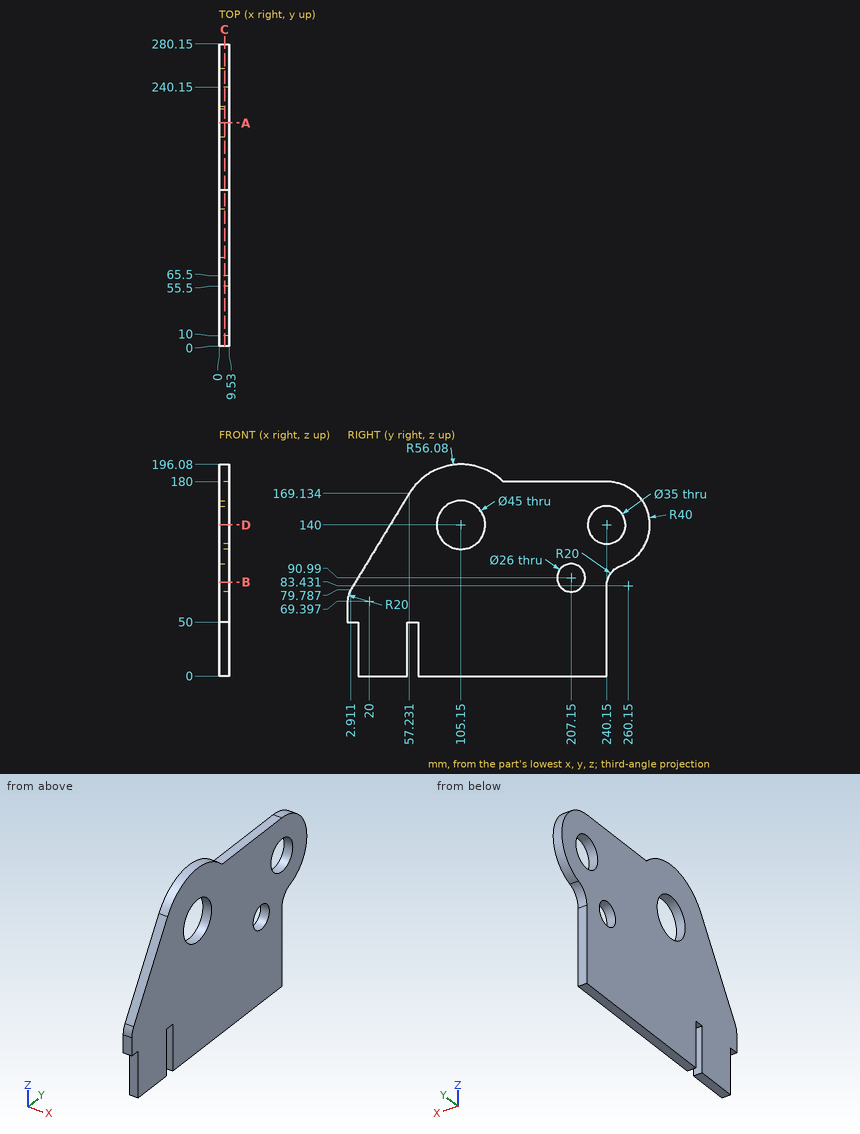
Answer from the drawing. Dimensions are ordinates in mm from the lowest x, y and z of the part. Coordinates: 2 decimals unless noted, no trailing zeros. Write each loop counter-clockwise with the first axis right and the second up, starting at its lowest first coordinate (ties: lowest second). Pieces come first, ordered by that corner, then holes. Notation, with made-up numbers: M -30.75,61 L 21.25,61 A34 cw 21.25,94 Z; hole C 47.5,-10.75 d5. An arc over 180 degrees is marked long. Use a Markdown table: item, result.
Q1. The part is cut by section D-D, the plane z = 140. Write down the section's boundary in (x, y).
Answer block:
| item | result |
|---|---|
| outline | M 0,39.52 L 9.53,39.52 L 9.53,82.65 L 0,82.65 Z; M 0,127.65 L 9.53,127.65 L 9.53,222.65 L 0,222.65 Z; M 0,257.65 L 9.53,257.65 L 9.53,280.15 L 0,280.15 Z |
Q2. Each of these flat-tipped pins is pushed along its axis until it touches: pin 1 Ø4 at (x, z) = (8, 164) entering from +Y; pin 2 Ø5 at (x, y) = (4.5, 61.5) entering from -Z; pin 3 Ø5 at (x, z) = (5, 25) entering from +Y. Where does it stop, or does it pass through?
Answer block:
| item | result |
|---|---|
| pin 1 | stops at y = 273.56 |
| pin 2 | stops at z = 50 |
| pin 3 | stops at y = 240.15 |
Q3. The part is cut by section A-A, the plane y = 207.15. Write down the section's boundary in (x, z), then the cut area to 3 significant figures.
Answer block:
| item | result |
|---|---|
| outline | M 0,0 L 9.53,0 L 9.53,77.99 L 0,77.99 Z; M 0,103.99 L 9.53,103.99 L 9.53,180 L 0,180 Z |
| area | 1,470 mm2 |
Q4. The part is cut by section C-C, the plane x = 5. Write down the section's boundary in (y, z).
Answer block:
| item | result |
|---|---|
| outline | M 0,50 L 10,50 L 10,0 L 55.5,0 L 55.5,50 L 65.5,50 L 65.5,0 L 240.15,0 L 240.15,83.43 A20 cw 253.48,102.29 A40 ccw 240.15,180 L 144.46,180 A56.08 ccw 57.23,169.13 L 2.91,79.79 A20 ccw 0,69.4 Z; hole C 105.15,140 d45; hole C 207.15,90.99 d26; hole C 240.15,140 d35 |
Q5. Straight lines are drawn through the part: L1, parallel to Y at x = 8, z = 134 (1 decimal); L2, parallel to Y at x = 4.75, z = 142 (1 decimal); L3, parallel to Y at x = 4, z = 10. For each, find the intervals that lie inside material, in ascending order. Write a range as [from, to].
Answer block:
| item | result |
|---|---|
| L1 | y = [35.9, 83.5], [126.8, 223.7], [256.6, 279.7] |
| L2 | y = [40.7, 82.7], [127.6, 222.8], [257.5, 280.1] |
| L3 | y = [10, 55.5], [65.5, 240.15] |
Q6. The part is cut by section B-B, the plane z = 87. Write down the section's boundary in (x, y) (1 decimal).
Answer block:
| item | result |
|---|---|
| outline | M 0,7.3 L 9.5,7.3 L 9.5,194.8 L 0,194.8 Z; M 0,219.5 L 9.5,219.5 L 9.5,240.5 L 0,240.5 Z |
